Check sheet for the drawn part. Datum: minimum x, y, z corner. Units: mm. A direction names the side the tool comes from. Give positions to 0.01 mm unless a question says otherwise; leave off trailing zeros. Write each loop counter-clockwise with the first axis right and the second up, starting at its lowest first coordinate (ties: lowest second). Pieces come first, ordered by that corner, then holes. Notation, with made-up numbers: M -19,72.5 L 2,72.5 A32 ccw 2,101.5 Z; hole C 72.5,49 d1. An arc over 180 degrees is marked long. Use CSV: the item, a comma, the result in double quotes. Start each with the question number.
1. Cross-section at B-B, the plane z = 0.65. Enter the section's corners in (x, y), and give its area (3 significant figures).
2. Access from +Z, -Z, +X, -X, +Y, -Y to the whole of each face (thin tool, end or side, straight path). Record for the marked faces 1 and 2.
3. Cross-section at A-A, the plane y = 45. Enter the section's corners in (x, z), and give its area (3 significant figures).
4. Depth check by flat-ended pin: P1, Ø5, axis at x = 14, y = 9, coming from the -Z side. Enter the tip coordinate at first touch or a pass-through.
5. Scan lines: line 1 (Y direction, x = 5, z = 1.8); line 2 (X direction, y = 5, z = 2.25); line 3 (X direction, y = 11.5, z = 1.1). Record each from-to range of solid material in increasing order.
6. Cross-section at D-D, the plane y = 25. Enter the section's corners in (x, z), and give its area (3 significant figures).
7. Cross-section at C-C, the plane x = 21. Enter the section's corners in (y, z).
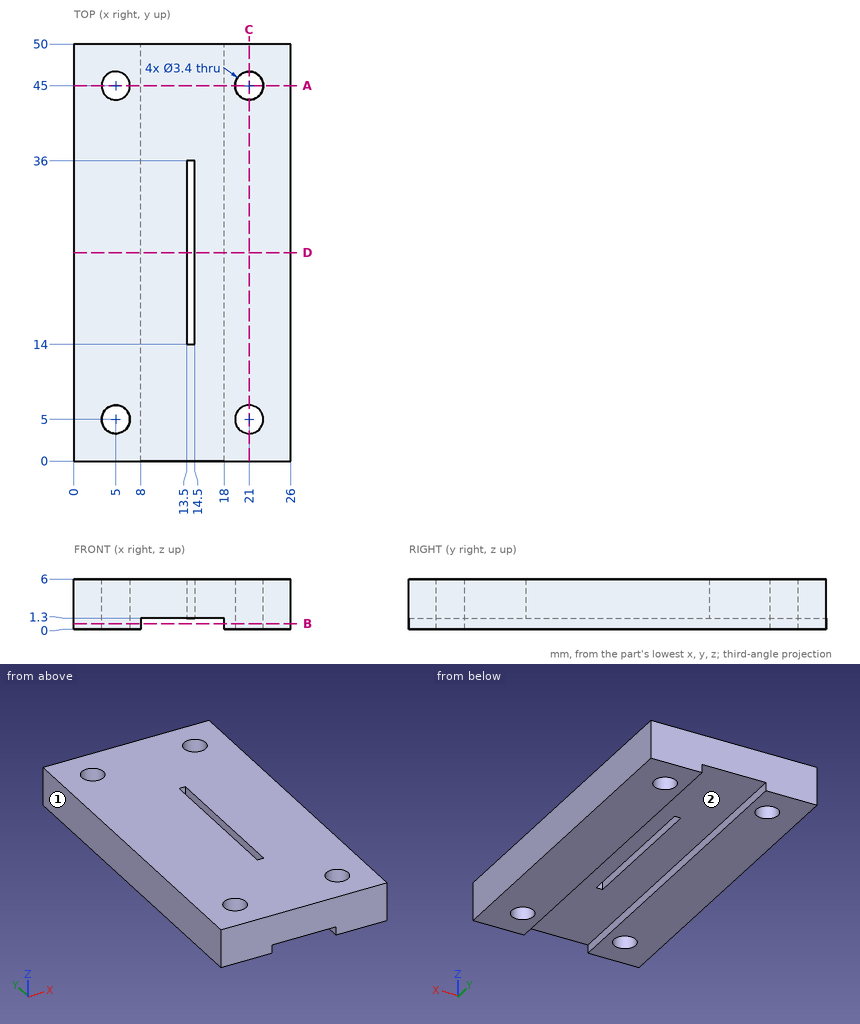
Worked answers:
1,outline,"M 0,0 L 8,0 L 8,50 L 0,50 Z; M 18,0 L 26,0 L 26,50 L 18,50 Z; hole C 5,5 d3.4; hole C 5,45 d3.4; hole C 21,5 d3.4; hole C 21,45 d3.4"
1,area,"764 mm^2"
2,face 1,"+Z, -Z, -X, +Y, -Y"
2,face 2,"-Z, +Y, -Y"
3,outline,"M 0,0 L 3.3,0 L 3.3,6 L 0,6 Z; M 6.7,0 L 8,0 L 8,1.3 L 18,1.3 L 18,0 L 19.3,0 L 19.3,6 L 6.7,6 Z; M 22.7,0 L 26,0 L 26,6 L 22.7,6 Z"
3,area,"102 mm^2"
4,P1,"stops at z = 1.3"
5,line 1,"y = 0 to 3.3, 6.7 to 43.3, 46.7 to 50"
5,line 2,"x = 0 to 3.3, 6.7 to 19.3, 22.7 to 26"
5,line 3,"x = 0 to 8, 18 to 26"
6,outline,"M 0,0 L 8,0 L 8,1.3 L 13.5,1.3 L 13.5,6 L 0,6 Z; M 14.5,1.3 L 18,1.3 L 18,0 L 26,0 L 26,6 L 14.5,6 Z"
6,area,"138 mm^2"
7,outline,"M 0,0 L 3.3,0 L 3.3,6 L 0,6 Z; M 6.7,0 L 43.3,0 L 43.3,6 L 6.7,6 Z; M 46.7,0 L 50,0 L 50,6 L 46.7,6 Z"
